Input: dimensioned drawing with shaded views. Units: mm. Origin: part minimum x, y, z. A direction names the side the tool comes from. Coordinates: 2 decimals unless noted, no trailing zeros. Loops run counter-clockwise (first coordinate to the right, second up) from the corner with the lowest first, then second, coordinate; pieces in that order, holes last. Notation, with made-up numbers: (-16, -28) - (22, -28) arc R8 ccw to (22, -17) - close; hole circle Ø3 at (8, 57). An arc over 180 degrees is marked (long way). Use one line per item in the form item = value. Start each with the question number.
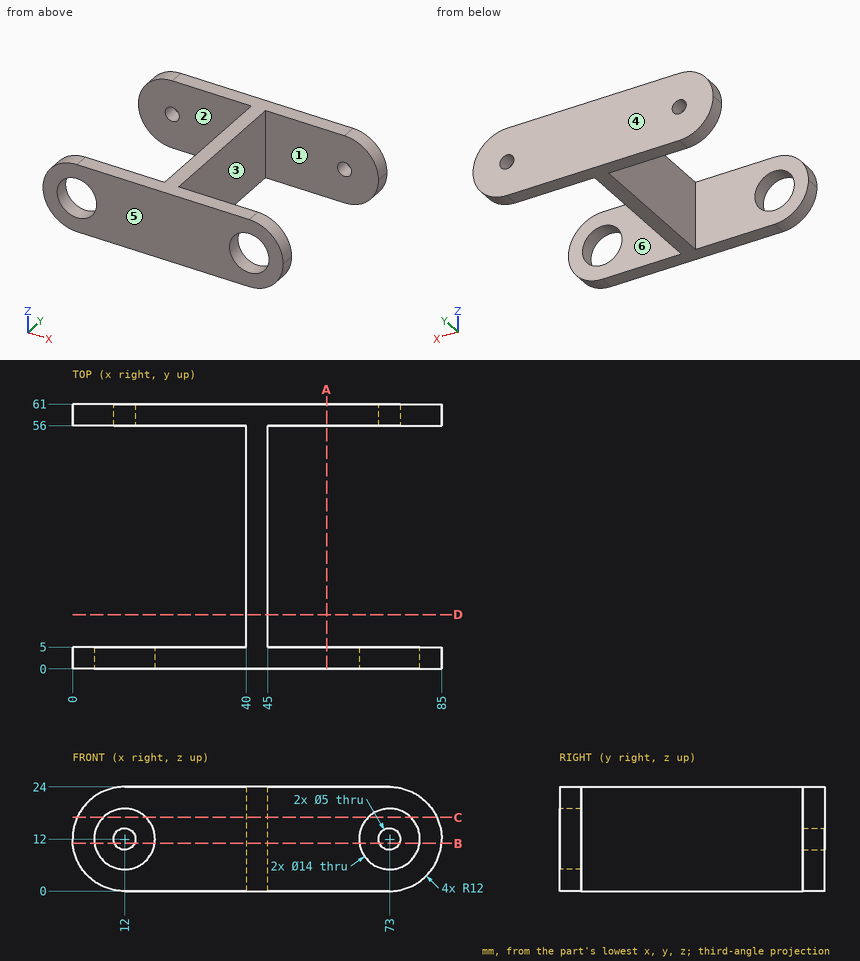
(1) Cut plane B-B, the plane z = 11. Output: boundary loops of the cut face in (x, y), plus the area to 3 significant figures.
(2) Mould query, pull axis Y, two halves, no side actions, for the marked faces 3, 4, 5 and 6. Classes: +Y half, -Y half, draft (parallel to the pull), parting line (faces both ways), or undercut.
(3) Material intervals for line 1 (Z direction, x = 12, y = 2.05); line 2 (Y direction, x = 34, z = 7.75); line 3 (Z direction, x = 73, y = 58), sorted ascending.
(4) Cut plane D-D, the plane y = 12.5. Output: boundary loops of the cut face in (x, z), plus the area to 3 significant figures.
(5) Access query for the marked faces 1 and 2. Directions: +Z, -Z, +X, -X, +Y, -Y. A direction counts if a zero-diameter tool reaches every point of the face in a straight line with its end or side. Return the directions, or none.
(6) Contact query for flat-ended pins moving along their axis: pin 1 (12 mm diameter, centred on y = 10.5, z = 17.5, fed in from +X); pin 2 (12.5 mm diameter, centred on x = 12, z = 12, fed in from -Y); pin 3 (8 mm diameter, centred on y = 41.5, z = 5.5, fed in from -X); pin 4 (3 mm diameter, centred on x = 73, z = 12, fed in from -Y). Output: stop coordinate, or through.
(7) Cut plane A-A, the plane x = 58.5. Output: boundary loops of the cut face in (y, z).
(8) Cut plane C-C, the plane z = 17. Output: boundary loops of the cut face in (x, y), plus the area to 3 significant figures.
Recorded:
q1.outline = (0.04, 0) - (5.07, 0) - (5.07, 5) - (0.04, 5) - close; (0.04, 56) - (9.71, 56) - (9.71, 61) - (0.04, 61) - close; (14.29, 56) - (40, 56) - (40, 5) - (18.93, 5) - (18.93, 0) - (66.07, 0) - (66.07, 5) - (45, 5) - (45, 56) - (70.71, 56) - (70.71, 61) - (14.29, 61) - close; (75.29, 56) - (84.96, 56) - (84.96, 61) - (75.29, 61) - close; (79.93, 0) - (84.96, 0) - (84.96, 5) - (79.93, 5) - close
q1.area = 920 mm²
q2.face_3 = undercut
q2.face_4 = +Y half
q2.face_5 = -Y half
q2.face_6 = undercut
q3.line_1 = 0 to 5, 19 to 24
q3.line_2 = 0 to 5, 56 to 61
q3.line_3 = 0 to 9.5, 14.5 to 24
q4.outline = (40, 0) - (45, 0) - (45, 24) - (40, 24) - close
q4.area = 120 mm²
q5.face_1 = +Z, -Z, +X
q5.face_2 = +Z, -Z, -X
q6.pin_1 = 84.59
q6.pin_2 = 56
q6.pin_3 = 40
q6.pin_4 = through
q7.outline = (0, 0) - (5, 0) - (5, 24) - (0, 24) - close; (56, 0) - (61, 0) - (61, 24) - (56, 24) - close
q8.outline = (1.09, 0) - (7.1, 0) - (7.1, 5) - (1.09, 5) - close; (1.09, 56) - (40, 56) - (40, 5) - (16.9, 5) - (16.9, 0) - (68.1, 0) - (68.1, 5) - (45, 5) - (45, 56) - (83.91, 56) - (83.91, 61) - (1.09, 61) - close; (77.9, 0) - (83.91, 0) - (83.91, 5) - (77.9, 5) - close
q8.area = 985 mm²
